For this review, take the finished solid that the model builds, in its own axes (mm). A direction names the side the tool comes from. Round coordinates to 2 decimals unless told otherwise and drop trailing zeros. Answer as a JSON object with one key per item and string values.
from build123d import *

# Parameters (mm, degrees)
SKETCH2_W           = 900
SKETCH2_H           = 300
BOSS_EXTRUDE1_DEPTH = 6.35
CUT_EXTRUDE1_DEPTH  = 6.35
SKETCH4_R           = 3.5
CUT_EXTRUDE2_DEPTH  = 949.704549636
CUT_EXTRUDE3_DEPTH  = 10


with BuildPart() as part:
    # Sketch2 → Boss-Extrude1 (new body)
    with BuildSketch(Plane.XY):
        with Locations((450, 150)):
            Rectangle(SKETCH2_W, SKETCH2_H)
    extrude(amount=BOSS_EXTRUDE1_DEPTH)

    # Sketch3 → Cut-Extrude1 (cut)
    with BuildSketch(Plane.XY.offset(6.35)):
        with BuildLine():
            Line((443.65, 210), (443.65, 260))
            ThreePointArc((443.65, 260), (450, 266.35), (456.35, 260))
            Line((456.35, 260), (456.35, 210))
            ThreePointArc((456.35, 210), (450, 203.65), (443.65, 210))
        make_face()
        with BuildLine():
            Line((481.35, 210), (481.35, 260))
            ThreePointArc((481.35, 260), (475, 266.35), (468.65, 260))
            Line((468.65, 260), (468.65, 210))
            ThreePointArc((468.65, 210), (475, 203.65), (481.35, 210))
        make_face()
        with BuildLine():
            Line((506.35, 210), (506.35, 260))
            ThreePointArc((506.35, 260), (500, 266.35), (493.65, 260))
            Line((493.65, 260), (493.65, 210))
            ThreePointArc((493.65, 210), (500, 203.65), (506.35, 210))
        make_face()
        with BuildLine():
            Line((531.35, 210), (531.35, 260))
            ThreePointArc((531.35, 260), (525, 266.35), (518.65, 260))
            Line((518.65, 260), (518.65, 210))
            ThreePointArc((518.65, 210), (525, 203.65), (531.35, 210))
        make_face()
        with BuildLine():
            Line((556.35, 210), (556.35, 260))
            ThreePointArc((556.35, 260), (550, 266.35), (543.65, 260))
            Line((543.65, 260), (543.65, 210))
            ThreePointArc((543.65, 210), (550, 203.65), (556.35, 210))
        make_face()
        with BuildLine():
            Line((581.35, 210), (581.35, 260))
            ThreePointArc((581.35, 260), (575, 266.35), (568.65, 260))
            Line((568.65, 260), (568.65, 210))
            ThreePointArc((568.65, 210), (575, 203.65), (581.35, 210))
        make_face()
        with BuildLine():
            Line((606.35, 210), (606.35, 260))
            ThreePointArc((606.35, 260), (600, 266.35), (593.65, 260))
            Line((593.65, 260), (593.65, 210))
            ThreePointArc((593.65, 210), (600, 203.65), (606.35, 210))
        make_face()
        with BuildLine():
            Line((631.35, 210), (631.35, 260))
            ThreePointArc((631.35, 260), (625, 266.35), (618.65, 260))
            Line((618.65, 260), (618.65, 210))
            ThreePointArc((618.65, 210), (625, 203.65), (631.35, 210))
        make_face()
        with BuildLine():
            Line((656.35, 210), (656.35, 260))
            ThreePointArc((656.35, 260), (650, 266.35), (643.65, 260))
            Line((643.65, 260), (643.65, 210))
            ThreePointArc((643.65, 210), (650, 203.65), (656.35, 210))
        make_face()
        with BuildLine():
            Line((681.35, 210), (681.35, 260))
            ThreePointArc((681.35, 260), (675, 266.35), (668.65, 260))
            Line((668.65, 260), (668.65, 210))
            ThreePointArc((668.65, 210), (675, 203.65), (681.35, 210))
        make_face()
        with BuildLine():
            Line((706.35, 210), (706.35, 260))
            ThreePointArc((706.35, 260), (700, 266.35), (693.65, 260))
            Line((693.65, 260), (693.65, 210))
            ThreePointArc((693.65, 210), (700, 203.65), (706.35, 210))
        make_face()
        with BuildLine():
            Line((731.35, 210), (731.35, 260))
            ThreePointArc((731.35, 260), (725, 266.35), (718.65, 260))
            Line((718.65, 260), (718.65, 210))
            ThreePointArc((718.65, 210), (725, 203.65), (731.35, 210))
        make_face()
        with BuildLine():
            Line((756.35, 210), (756.35, 260))
            ThreePointArc((756.35, 260), (750, 266.35), (743.65, 260))
            Line((743.65, 260), (743.65, 210))
            ThreePointArc((743.65, 210), (750, 203.65), (756.35, 210))
        make_face()
        with BuildLine():
            Line((781.35, 210), (781.35, 260))
            ThreePointArc((781.35, 260), (775, 266.35), (768.65, 260))
            Line((768.65, 260), (768.65, 210))
            ThreePointArc((768.65, 210), (775, 203.65), (781.35, 210))
        make_face()
        with BuildLine():
            Line((806.35, 210), (806.35, 260))
            ThreePointArc((806.35, 260), (800, 266.35), (793.65, 260))
            Line((793.65, 260), (793.65, 210))
            ThreePointArc((793.65, 210), (800, 203.65), (806.35, 210))
        make_face()
        with BuildLine():
            Line((831.35, 210), (831.35, 260))
            ThreePointArc((831.35, 260), (825, 266.35), (818.65, 260))
            Line((818.65, 260), (818.65, 210))
            ThreePointArc((818.65, 210), (825, 203.65), (831.35, 210))
        make_face()
        with BuildLine():
            Line((431.35, 210), (431.35, 260))
            ThreePointArc((431.35, 260), (425, 266.35), (418.65, 260))
            Line((418.65, 260), (418.65, 210))
            ThreePointArc((418.65, 210), (425, 203.65), (431.35, 210))
        make_face()
        with BuildLine():
            Line((406.35, 210), (406.35, 260))
            ThreePointArc((406.35, 260), (400, 266.35), (393.65, 260))
            Line((393.65, 260), (393.65, 210))
            ThreePointArc((393.65, 210), (400, 203.65), (406.35, 210))
        make_face()
        with BuildLine():
            Line((381.35, 210), (381.35, 260))
            ThreePointArc((381.35, 260), (375, 266.35), (368.65, 260))
            Line((368.65, 260), (368.65, 210))
            ThreePointArc((368.65, 210), (375, 203.65), (381.35, 210))
        make_face()
        with BuildLine():
            Line((356.35, 210), (356.35, 260))
            ThreePointArc((356.35, 260), (350, 266.35), (343.65, 260))
            Line((343.65, 260), (343.65, 210))
            ThreePointArc((343.65, 210), (350, 203.65), (356.35, 210))
        make_face()
        with BuildLine():
            Line((331.35, 210), (331.35, 260))
            ThreePointArc((331.35, 260), (325, 266.35), (318.65, 260))
            Line((318.65, 260), (318.65, 210))
            ThreePointArc((318.65, 210), (325, 203.65), (331.35, 210))
        make_face()
        with BuildLine():
            Line((306.35, 210), (306.35, 260))
            ThreePointArc((306.35, 260), (300, 266.35), (293.65, 260))
            Line((293.65, 260), (293.65, 210))
            ThreePointArc((293.65, 210), (300, 203.65), (306.35, 210))
        make_face()
        with BuildLine():
            Line((281.35, 210), (281.35, 260))
            ThreePointArc((281.35, 260), (275, 266.35), (268.65, 260))
            Line((268.65, 260), (268.65, 210))
            ThreePointArc((268.65, 210), (275, 203.65), (281.35, 210))
        make_face()
        with BuildLine():
            Line((256.35, 210), (256.35, 260))
            ThreePointArc((256.35, 260), (250, 266.35), (243.65, 260))
            Line((243.65, 260), (243.65, 210))
            ThreePointArc((243.65, 210), (250, 203.65), (256.35, 210))
        make_face()
        with BuildLine():
            Line((231.35, 210), (231.35, 260))
            ThreePointArc((231.35, 260), (225, 266.35), (218.65, 260))
            Line((218.65, 260), (218.65, 210))
            ThreePointArc((218.65, 210), (225, 203.65), (231.35, 210))
        make_face()
        with BuildLine():
            Line((206.35, 210), (206.35, 260))
            ThreePointArc((206.35, 260), (200, 266.35), (193.65, 260))
            Line((193.65, 260), (193.65, 210))
            ThreePointArc((193.65, 210), (200, 203.65), (206.35, 210))
        make_face()
        with BuildLine():
            Line((181.35, 210), (181.35, 260))
            ThreePointArc((181.35, 260), (175, 266.35), (168.65, 260))
            Line((168.65, 260), (168.65, 210))
            ThreePointArc((168.65, 210), (175, 203.65), (181.35, 210))
        make_face()
        with BuildLine():
            Line((156.35, 210), (156.35, 260))
            ThreePointArc((156.35, 260), (150, 266.35), (143.65, 260))
            Line((143.65, 260), (143.65, 210))
            ThreePointArc((143.65, 210), (150, 203.65), (156.35, 210))
        make_face()
        with BuildLine():
            Line((131.35, 210), (131.35, 260))
            ThreePointArc((131.35, 260), (125, 266.35), (118.65, 260))
            Line((118.65, 260), (118.65, 210))
            ThreePointArc((118.65, 210), (125, 203.65), (131.35, 210))
        make_face()
        with BuildLine():
            Line((106.35, 210), (106.35, 260))
            ThreePointArc((106.35, 260), (100, 266.35), (93.65, 260))
            Line((93.65, 260), (93.65, 210))
            ThreePointArc((93.65, 210), (100, 203.65), (106.35, 210))
        make_face()
        with BuildLine():
            Line((81.35, 210), (81.35, 260))
            ThreePointArc((81.35, 260), (75, 266.35), (68.65, 260))
            Line((68.65, 260), (68.65, 210))
            ThreePointArc((68.65, 210), (75, 203.65), (81.35, 210))
        make_face()
    extrude(amount=-CUT_EXTRUDE1_DEPTH, mode=Mode.SUBTRACT)

    # Sketch4 → Cut-Extrude2 (cut, through all)
    with BuildSketch(Plane.XY.offset(6.35)):
        with Locations((12.5, 50)):
            Circle(SKETCH4_R)
        with Locations((12.5, 250)):
            Circle(SKETCH4_R)
        with Locations((450, 287.5)):
            Circle(SKETCH4_R)
        with Locations((800, 287.5)):
            Circle(SKETCH4_R)
        with Locations((100, 287.5)):
            Circle(SKETCH4_R)
        with Locations(Location((887.5, 50, 0), (0, 0, 180))):
            Circle(SKETCH4_R)
        with Locations(Location((887.5, 250, 0), (0, 0, 180))):
            Circle(SKETCH4_R)
        with Locations(Location((800, 12.5, 0), (0, 0, 180))):
            Circle(SKETCH4_R)
        with Locations(Location((450, 12.5, 0), (0, 0, 180))):
            Circle(SKETCH4_R)
        with Locations(Location((100, 12.5, 0), (0, 0, 180))):
            Circle(SKETCH4_R)
    extrude(amount=-CUT_EXTRUDE2_DEPTH, mode=Mode.SUBTRACT)

    # Sketch5 → Cut-Extrude3 (cut)
    with BuildSketch(Plane(origin=(0, 0, 0), x_dir=(-1, 0, 0), z_dir=(0, 0, -1))):
        with BuildLine():
            Line((-812.5, 90), (-687.5, 90))
            ThreePointArc((-687.5, 90), (-662.5, 65), (-687.5, 40))
            Line((-687.5, 40), (-812.5, 40))
            ThreePointArc((-812.5, 40), (-837.5, 65), (-812.5, 90))
        make_face()
    extrude(amount=-CUT_EXTRUDE3_DEPTH, mode=Mode.SUBTRACT)


solid = part.part
1) Mouldability with a two-part tool opening along Y and no side actions: class faces 3 (the flat face through (444, 152, 6.35)), 4 (the cylindrical face through (837.494, 64.45, 3.131)) as +Y half, -Y half, draft (parallel to the pull), parting line (faces both ways), or undercut.
Geometry check:
{"face 3": "draft", "face 4": "undercut"}
2) Add section A-A on z = 1. State how many separate pieces and enclosed holes the cut face has, and give its area (3 significant figures).
Geometry check:
{"separate pieces": "1", "enclosed holes": "42", "area": "238,000 mm²"}
3) Machinability: for faces 1 (the cylindrical face through (662.506, 65.55, 3.131)), 2 (the flat face through (444, 152, 0)), which of the approach directions +Z, -Z, +X, -X, +Y, -Y give a long, thin tool a straight path to every point of the face, cutting with its end or side? Answer none if there is none.
Geometry check:
{"face 1": "+Z, -Z", "face 2": "-Z, +X, -X, +Y, -Y"}
4) Insertion check: P1, Ø3, axis at y = 232.5, z = 3.5, coming from the -X side. The pin has a flat end and moves straight along its axis. Give the tip position at first contact, or say it passes through.
Geometry check:
{"P1": "stops at x = 0"}
5) For L1, parallel to Y at x = 12.5, z = 4.75; L2, parallel to Y at x = 100, z = 5; L3, parallel to X at y = 287.5, z = 3, list the stretches that pass through material, from the lowest coordinate up.
Geometry check:
{"L1": "y = 0 to 46.5, 53.5 to 246.5, 253.5 to 300", "L2": "y = 0 to 9, 16 to 203.65, 266.35 to 284, 291 to 300", "L3": "x = 0 to 96.5, 103.5 to 446.5, 453.5 to 796.5, 803.5 to 900"}
